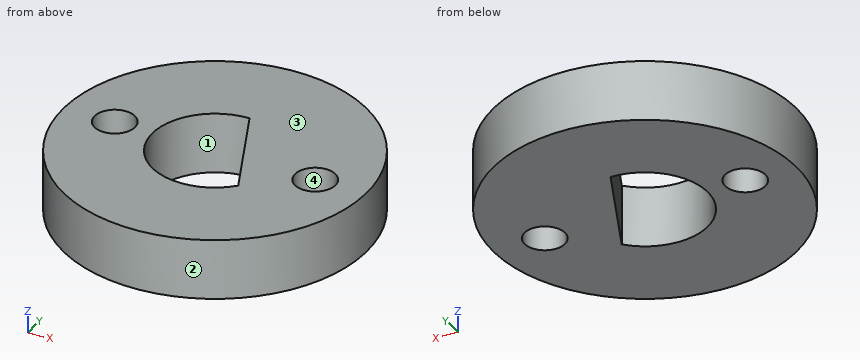
from build123d import *

# Parameters (mm, degrees)
SKETCH1_R             = 7.5
BOSS_EXTRUDE1_DEPTH   = 3
CUT_EXTRUDE1_DEPTH    = 3
F_2_0MM_DOWEL_HOLE1_D = 2


with BuildPart() as part:
    # Sketch1 → Boss-Extrude1 (new body)
    with BuildSketch(Plane.XY):
        Circle(SKETCH1_R)
    extrude(amount=BOSS_EXTRUDE1_DEPTH)

    # Sketch2 → Cut-Extrude1 (cut)
    with BuildSketch(Plane.XY.offset(3)):
        with BuildLine():
            Line((0, 3.1), (2.308854941, -2.068620038))
            ThreePointArc((2.308854941, -2.068620038), (-2.830434783, -1.264372944), (0, 3.1))
        make_face()
    extrude(amount=-CUT_EXTRUDE1_DEPTH, mode=Mode.SUBTRACT)

    # Ø2.0mm Dowel Hole1 (through all)
    with Locations(Plane.XY.offset(3)):
        with Locations((-5, 0), (5, 0)):
            Hole(F_2_0MM_DOWEL_HOLE1_D / 2)


solid = part.part
Read the model definition and answer for the solid it produces. Units are mm, in the model's axes. Face numbers are marked on the shaded views. Coordinates: 2 decimals unless noted, no trailing zeros. Write each loop counter-clockwise with the first axis right and the second up, starting at its lowest first coordinate (ties: lowest second). Pieces come first, ordered by that corner, then holes. Notation, with made-up numbers: (80, 78.25) -> (108, 78.25) arc R35 cw to (108, 110.25) -> close; hole circle Ø3 at (-36, -11.75). An arc over 180 degrees is marked (long way). Return JSON: item names as keys, results as strings.
(1) The part is cut by section D-D on z = 2.4. Give the vertices of the cut face in (x, y), then the cut area to 3 significant figures.
Answers below:
{"outline": "circle Ø15 at (0, 0); hole circle Ø2 at (-5, 0); hole (0, 3.1) arc R3.1 ccw (long way) to (2.31, -2.07) -> close; hole circle Ø2 at (5, 0)", "area": "148 mm^2"}
(2) Each of these flat-tipped pins is pushed along its axis until it touches: P1, Ø1, axis at y = -4, z = 1, coming from the -X side; P2, Ø1, axis at x = -2, z = 1, coming from the +Y side; P3, Ø1.6, axis at x = 5, y = 0, coming from the -Z side. Where does it stop, or does it pass through?
Answers below:
{"P1": "x = -6.63", "P2": "y = 7.35", "P3": "through"}
(3) The part is cut by section C-C on y = 2. Give the vertices of the cut face in (x, z), then the cut area to 3 significant figures.
Answers below:
{"outline": "(-7.23, 0) -> (-2.37, 0) -> (-2.37, 3) -> (-7.23, 3) -> close; (0.49, 0) -> (7.23, 0) -> (7.23, 3) -> (0.49, 3) -> close", "area": "34.8 mm^2"}
(4) For a pull along Y with two mould halves and no side action, classify the marked faces 1, 2, 3 and 4 as pulls with the +Y half, pulls with the -Y half, needs draft (parallel to the pull), parting line crosses it, or undercut.
Answers below:
{"face 1": "undercut", "face 2": "parting line crosses it", "face 3": "needs draft", "face 4": "undercut"}
(5) The part is cut by section A-A on x = -2.5. Give the vertices of the cut face in (y, z).
Answers below:
{"outline": "(-7.07, 0) -> (-1.83, 0) -> (-1.83, 3) -> (-7.07, 3) -> close; (1.83, 0) -> (7.07, 0) -> (7.07, 3) -> (1.83, 3) -> close"}
(6) The part is cut by section B-B on y = 0. Give the vertices of the cut face in (x, z), then the cut area to 3 significant figures.
Answers below:
{"outline": "(-7.5, 0) -> (-6, 0) -> (-6, 3) -> (-7.5, 3) -> close; (-4, 0) -> (-3.1, 0) -> (-3.1, 3) -> (-4, 3) -> close; (1.38, 0) -> (4, 0) -> (4, 3) -> (1.38, 3) -> close; (6, 0) -> (7.5, 0) -> (7.5, 3) -> (6, 3) -> close", "area": "19.5 mm^2"}
(7) Consider line 1 along X through (y, z) = (-4.5, 0.8); line 2 along Y through (x, z) = (4.75, 1.95); line 3 along X through (y, z) = (-2, 1.7). Determine where each line is inside the solid, lowest interval first. Write a range as from..to.
Answers below:
{"line 1": "-6..6", "line 2": "-5.8..-0.97, 0.97..5.8", "line 3": "-7.23..-2.37, 2.28..7.23"}
